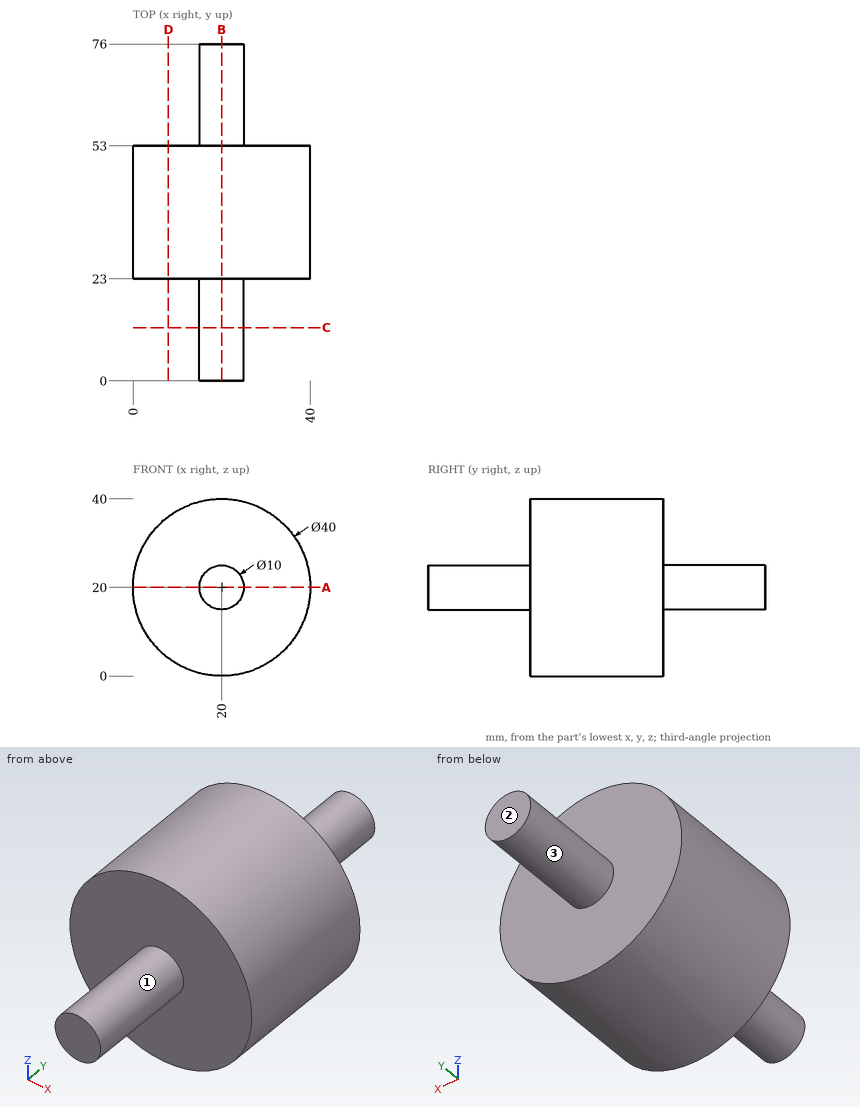
Geometry check sheet. Reference: drawing and pictorial views, mm from the part's lowest x, y, z. A direction names the side the tool comes from. Round coordinates to 2 decimals unless told otherwise and drop trailing zeros. Write each loop counter-clockwise with the first axis right and the second up, starting at its lowest first coordinate (ties: lowest second). Pieces come first, ordered by that corner, then holes. Notation, with made-up numbers: (55.25, 62) -> (60.25, 62) arc R15 cw to (60.25, 89) -> close; hole circle Ø8 at (22, -23.75). An arc over 180 degrees is marked (long way). Put each result on its own line as item: value.
1) Cross-section at B-B, the plane x = 20. Enter the section's corners in (y, z).
Recorded:
outline: (0, 15) -> (23, 15) -> (23, 0) -> (53, 0) -> (53, 15) -> (76, 15) -> (76, 25) -> (53, 25) -> (53, 40) -> (23, 40) -> (23, 25) -> (0, 25) -> close
2) Thickness scan on probe 1 along Z at (x, y) = (20, 59); probe 2 along Y at (x, z) = (35.5, 16.5). Record the ranges inside material, lowest first. Write a range as from..to.
Recorded:
probe 1: z = 15..25
probe 2: y = 23..53
3) Access from +Z, -Z, +X, -X, +Y, -Y to the whole of each face (thin tool, end or side, straight path). Record for the marked faces 1, 2 and 3.
Recorded:
face 1: -Y
face 2: +Z, -Z, +X, -X, +Y
face 3: +Y
4) Depth check by flat-ended pin: P1, Ø20, axis at x = 27, z = 28.5, coming from the -Y side; P2, Ø1, axis at x = 26, z = 11, coming from the -Y side; P3, Ø12, axis at x = 27.5, y = 55, coming from the +Z side; P4, Ø12, axis at y = 26.5, z = 29.5, coming from the +X side. Enter the tip coordinate at first touch or a pass-through.
Recorded:
P1: stops at y = 0
P2: stops at y = 23
P3: stops at z = 39.91
P4: stops at x = 39.69
5) Cross-section at D-D, the plane x = 8. Enter the section's corners in (y, z), plus the area to 3 significant figures.
Recorded:
outline: (23, 4) -> (53, 4) -> (53, 36) -> (23, 36) -> close
area: 960 mm2
6) Cross-section at C-C, the plane y = 12. Enter the section's corners in (x, z), plus the area to 3 significant figures.
Recorded:
outline: circle Ø10 at (20, 20)
area: 78.5 mm2
7) Cross-section at A-A, the plane z = 20. Enter the section's corners in (x, y).
Recorded:
outline: (0, 23) -> (15, 23) -> (15, 0) -> (25, 0) -> (25, 23) -> (40, 23) -> (40, 53) -> (25, 53) -> (25, 76) -> (15, 76) -> (15, 53) -> (0, 53) -> close
